Autodesk Inventor part; units mm, degrees
ref_plane "YZ Plane" through (0, 0, 0) normal (1, 0, 0) x (0, 1, 0)
ref_plane "XZ Plane" through (0, 0, 0) normal (0, 1, 0) x (-1, 0, 0)
ref_plane "XY Plane" through (0, 0, 0) normal (0, 0, 1) x (1, 0, 0)
sketch "Sketch1" plane through (0, 0, 0) normal (0, 0, 1) x (1, 0, 0)
  line L0 (-9.75, 17.5) -> (9.75, 17.5)
  line L1 (9.75, 17.5) -> (9.75, -17.5)
  line L2 (9.75, -17.5) -> (-9.75, -17.5)
  line L3 (-9.75, -17.5) -> (-9.75, 17.5)
  line L4 (-9.75, 17.5) -> (9.75, -17.5) construction
  line L5 (9.75, 17.5) -> (-9.75, -17.5) construction
  point P0 (0, 0)
  dimension "d0" = 19.5
  dimension "d1" = 35
extrude "Extrusion1" add sketch "Sketch1" along normal blind 7.9
sketch "Sketch2" plane through (0, 0, 7.9) normal (0, 0, 1) x (1, 0, 0)
  line L0 (-5, 10) -> (5, 10)
  line L1 (5, 10) -> (5, -10)
  line L2 (5, -10) -> (-5, -10)
  line L3 (-5, -10) -> (-5, 10)
  line L4 (-5, 10) -> (5, -10) construction
  line L5 (5, 10) -> (-5, -10) construction
  point P0 (0, 0)
  dimension "d4" = 10
  dimension "d5" = 20
hole "Hole1" at (-5, 10, 7.9) at (5, 10, 7.9) at (5, -10, 7.9) at (-5, -10, 7.9) direction (0, 0, -1) diameter 3.4 end through all countersink diameter 8 countersink angle 90
fillet "Fillet1" radius 5 4 edges at (9.75, -17.5, 3.95) (-9.75, -17.5, 3.95) (-9.75, 17.5, 3.95) (9.75, 17.5, 3.95)
properties part number "RailTab"
Build history of the part. All positions in model axes, mm. Give positions to 0.01 mm unless a question says otherwise; leave off trailing zeros. Loops run counter-clockwise (first coordinate to the right, second up) from the corner with the lowest first, then second, coordinate; pieces in that order, holes last. Notation, with made-up numbers: (8, 58) -> (33, 58) arc R11 cw to (33, 70) -> close; hole circle Ø3 at (-6.5, -19.75). An arc over 180 degrees is marked (long way). One line per question, with ' | ' between items. Start each with the question number.
1) Two-plate mould, pull along Y, no slides. Class faces 1 (the conical face through (4.29, -11.7, 5.74)), 2 (the flat face through (0, 17.5, 4)), 3 (the flat face through (-9.75, 0, 4)): released by +Y, released by -Y, zero draft, split by the parting line, or undercut.
2) Cut at D-D (x = 5.5). Count the separate pieces of the cut face and the enclosed holes in it, plus the area to 3 significant figures.
3) Probe L1, parallel to X at y = 10, z = 3.8; L2, parallel to Y at x = 5, z = 2.45; L3, parallel to X at y = 11.5, z = 3. List the from-to ranges inside material, lowest first.
4) Pin check, flat tips, straight feed: pin 1 (2 mm diameter, centred on x = -5, y = 10, fed in from +Z); pin 2 (4 mm diameter, centred on x = -5, y = -10, fed in from +Z). Stop position of each tip, or through.
5) Cut at B-B (z = 7.25). Give the cut face in (x, y), plus the area to 3 significant figures.
6) Cut at A-A (y = 10). Give the cut face in (x, z).
7) Cut at C-C (z = 3.5). Give the cut face in (x, y), plus the area to 3 significant figures.
Return value:
1) face 1: undercut | face 2: released by +Y | face 3: zero draft
2) separate pieces: 3 | enclosed holes: 0 | area: 213 mm^2
3) L1: -9.75 to -6.7, -3.3 to 3.3, 6.7 to 9.75 | L2: -17.49 to -11.7, -8.3 to 8.3, 11.7 to 17.49 | L3: -9.75 to -5.8, -4.2 to 4.2, 5.8 to 9.75
4) pin 1: through | pin 2: z = 5.9
5) outline: (-9.75, -12.5) arc R5 ccw to (-4.75, -17.5) -> (4.75, -17.5) arc R5 ccw to (9.75, -12.5) -> (9.75, 12.5) arc R5 ccw to (4.75, 17.5) -> (-4.75, 17.5) arc R5 ccw to (-9.75, 12.5) -> close; hole circle Ø6.7 at (-5, -10); hole circle Ø6.7 at (-5, 10); hole circle Ø6.7 at (5, -10); hole circle Ø6.7 at (5, 10) | area: 520 mm^2
6) outline: (-9.75, 0) -> (-6.7, 0) -> (-6.7, 5.6) -> (-9, 7.9) -> (-9.75, 7.9) -> close; (-3.3, 0) -> (3.3, 0) -> (3.3, 5.6) -> (1, 7.9) -> (-1, 7.9) -> (-3.3, 5.6) -> close; (6.7, 0) -> (9.75, 0) -> (9.75, 7.9) -> (9, 7.9) -> (6.7, 5.6) -> close
7) outline: (-9.75, -12.5) arc R5 ccw to (-4.75, -17.5) -> (4.75, -17.5) arc R5 ccw to (9.75, -12.5) -> (9.75, 12.5) arc R5 ccw to (4.75, 17.5) -> (-4.75, 17.5) arc R5 ccw to (-9.75, 12.5) -> close; hole circle Ø3.4 at (-5, -10); hole circle Ø3.4 at (-5, 10); hole circle Ø3.4 at (5, -10); hole circle Ø3.4 at (5, 10) | area: 625 mm^2
